Input: part model. Units: mm. Frame: model coordinates. A direction names the side the tool comes from. Give positions to 0.01 mm unless a question says otherwise; leave off trailing zeros. Write each loop counter-clockwise with the first axis right and the second up, starting at its lowest first coordinate (ties: lowest second). Pieces come first, ordered by that corner, then holes. Notation, with made-up numbers: (21, 65) - (52, 65) arc R33 cw to (52, 93) - close; hole circle Ø10 at (-21.75, 52). An arc over 180 degrees is marked (long way). Answer as CSV lines item,"result".
```python
from build123d import *

# Parameters (mm, degrees)
F0_W           = 12.7
F0_H           = 3.175
F1_DEPTH       = 6.35
F2_DEPTH       = 3.683
F4_DEPTH       = 30.48
F5_W           = 7.1628
F5_H           = 7.2898
F6_DEPTH       = 38.101
F3_W           = 6.731
F3_H           = 12.7
F7_DEPTH       = 11.43
F8_W           = 3.5814
F8_H           = 3.6449
F9_DEPTH       = 12.7
F11_DEPTH      = 11.43
F12_W          = 7.2898
F12_H          = 7.1628
F13_DEPTH      = 6.731
F13_DEPTH_BACK = 31.369
F14_W          = 7.2898
F14_H          = 7.1628
F15_DEPTH      = 6.731
F15_DEPTH_BACK = 31.369
F16_W          = 7.1628
F16_H          = 7.2898
F17_DEPTH      = 8.128
F18_DEPTH      = 8.128
F19_DEPTH      = 8.128
F20_W          = 11.43
F20_H          = 12.7
F20_W_2        = 7.1628
F20_H_2        = 7.2898
F21_DEPTH      = 8.128
F22_DEPTH      = 8.128
F23_DEPTH      = 8.128
F24_W          = 12.7
F24_H          = 11.43
F24_R          = 2.286
F25_DEPTH      = 2.032
F26_W          = 12.7
F26_H          = 11.43
F26_R          = 2.286
F27_DEPTH      = 2.032
F28_W          = 11.43
F28_H          = 12.7
F28_R          = 2.286
F29_DEPTH      = 2.032
F30_W          = 12.7
F30_H          = 11.43
F30_R          = 2.286
F31_DEPTH      = 2.032
F32_W          = 12.7
F32_H          = 11.43
F32_R          = 2.286
F33_DEPTH      = 2.032
F34_W          = 30.48
F34_H          = 12.7
F34_R          = 2.286
F35_DEPTH      = 2.032
F36_R          = 1.9533985806
F36_R_2        = 1.1294229331
F36_R_3        = 1.2624825339
F36_R_4        = 1.2356748077
F36_R_5        = 1.4795101848
F36_R_6        = 1.3424473069
F36_R_7        = 0.8820699454
F36_R_8        = 0.8709860762
F36_R_9        = 1.0254141301
F36_R_10       = 0.6987220166
F36_R_11       = 1.012521994
F36_W          = 3.4493412822
F36_H          = 0.7421383634
F36_W_2        = 3.1675938517
F36_H_2        = 1.3768810313
F36_W_3        = 3.0767889693
F36_H_3        = 1.3319775462
F37_DEPTH      = 0.508


with BuildPart() as f1:
    # F0 (on Front) → F1 (new body, symmetric)
    with BuildSketch(Plane.XZ):
        with BuildLine():
            Line((0, 3.175), (0, 0))
            Line((0, 0), (13.335, 0))
            ThreePointArc((13.335, 0), (19.6211792847, -2.6038207153), (22.225, -8.89))
            Line((22.225, -8.89), (22.225, -22.225))
            Line((22.225, -22.225), (25.4, -22.225))
            Line((25.4, -22.225), (25.4, 3.175))
            Line((25.4, 3.175), (0, 3.175))
        make_face()
        with BuildLine():
            Line((13.335, 0), (0, 0))
            Line((0, 0), (0, -3.556))
            Line((0, -3.556), (11.557, -3.556))
            ThreePointArc((11.557, -3.556), (16.5859434278, -5.6390565722), (18.669, -10.668))
            Line((18.669, -10.668), (18.669, -22.225))
            Line((18.669, -22.225), (22.225, -22.225))
            Line((22.225, -22.225), (22.225, -8.89))
            ThreePointArc((22.225, -8.89), (19.6211792847, -2.6038207153), (13.335, 0))
        make_face()
        with Locations((-6.35, 1.5875)):
            Rectangle(F0_W, F0_H)
        with BuildLine():
            Line((0, -3.556), (0, 0))
            Line((0, 0), (-12.7, 0))
            Line((-12.7, 0), (-12.7, -22.225))
            Line((-12.7, -22.225), (-5.969, -22.225))
            Line((-5.969, -22.225), (-5.969, -8.636))
            ThreePointArc((-5.969, -8.636), (-4.4811024484, -5.0438975516), (-0.889, -3.556))
            Line((-0.889, -3.556), (0, -3.556))
        make_face()
    extrude(amount=F1_DEPTH, both=True)

    # F0 (on Front) → F2 (cut, symmetric)
    with BuildSketch(Plane.XZ):
        with BuildLine():
            Line((13.335, 0), (0, 0))
            Line((0, 0), (0, -3.556))
            Line((0, -3.556), (11.557, -3.556))
            ThreePointArc((11.557, -3.556), (16.5859434278, -5.6390565722), (18.669, -10.668))
            Line((18.669, -10.668), (18.669, -22.225))
            Line((18.669, -22.225), (22.225, -22.225))
            Line((22.225, -22.225), (22.225, -8.89))
            ThreePointArc((22.225, -8.89), (19.6211792847, -2.6038207153), (13.335, 0))
        make_face()
        with BuildLine():
            Line((0, -3.556), (0, 0))
            Line((0, 0), (-12.7, 0))
            Line((-12.7, 0), (-12.7, -22.225))
            Line((-12.7, -22.225), (-5.969, -22.225))
            Line((-5.969, -22.225), (-5.969, -8.636))
            ThreePointArc((-5.969, -8.636), (-4.4811024484, -5.0438975516), (-0.889, -3.556))
            Line((-0.889, -3.556), (0, -3.556))
        make_face()
    extrude(amount=F2_DEPTH, both=True, mode=Mode.SUBTRACT)

    # F3 (on face) → F4 (join)
    with BuildSketch(Plane.XZ.offset(6.35)):
        Polygon((18.669, -10.668), (18.669, -22.225), (25.4, -22.225), (25.4, -9.525), (18.669, -9.525), align=None)
    extrude(amount=F4_DEPTH)

    # F5 (on face) → F6 (cut, through all)
    with BuildSketch(Plane.YZ.offset(25.4)):
        with Locations((-11.6205, -15.875)):
            Rectangle(F5_W, F5_H)
        with Locations((-21.1455, -15.875)):
            Rectangle(F5_W, F5_H)
        with Locations((-30.6705, -15.875)):
            Rectangle(F5_W, F5_H)
    extrude(amount=-F6_DEPTH, mode=Mode.SUBTRACT)

    # F3 (on face) → F7 (join)
    with BuildSketch(Plane.XZ.offset(6.35)):
        with Locations((-9.3345, -15.875)):
            Rectangle(F3_W, F3_H)
    extrude(amount=F7_DEPTH)

    # F8 (on face) → F9 (cut)
    with BuildSketch(Plane(origin=(-12.7, 0, 0), x_dir=(0, -1, 0), z_dir=(-1, 0, 0))):
        with Locations((13.4112, -14.05255)):
            Rectangle(F8_W, F8_H)
        with Locations((9.8298, -14.05255)):
            Rectangle(F8_W, F8_H)
        Polygon((15.2019, -19.5199), (15.2019, -15.875), (11.6205, -15.875), (8.0391, -15.875), (8.0391, -19.5199), align=None)
    extrude(amount=-F9_DEPTH, mode=Mode.SUBTRACT)

    # F10 (on face) → F11 (join, through all)
    with BuildSketch(Plane.XZ.offset(6.35)):
        Polygon((-5.969, -9.525), (-5.308761314, -8.3814330508), (5.689761314, -2.0314330508), (7.010238686, -2.0314330508), (18.008761314, -8.3814330508), (18.669, -9.525), (25.4, -9.525), (21.374261314, -2.5522160579), (10.375738686, 3.7977839421), (2.324261314, 3.7977839421), (-8.674261314, -2.5522160579), (-12.7, -9.525), align=None)
        Polygon((18.008761314, -23.3685669492), (7.010238686, -29.7185669492), (5.689761314, -29.7185669492), (-5.308761314, -23.3685669492), (-5.969, -22.225), (-12.7, -22.225), (-8.674261314, -29.1977839421), (2.324261314, -35.5477839421), (10.375738686, -35.5477839421), (21.374261314, -29.1977839421), (25.4, -22.225), (18.669, -22.225), align=None)
    extrude(amount=F11_DEPTH)

    # F12 (on face) → F13 (cut, two sides)
    with BuildSketch(Plane(origin=(2.3020766425, 0, -3.9873137078), x_dir=(0.8660254038, 0, 0.5), z_dir=(0.5, 0, -0.8660254038))) as f13_sk:
        with Locations((-2.438238686, 11.6205)):
            Rectangle(F12_W, F12_H)
    extrude(amount=-F13_DEPTH, mode=Mode.SUBTRACT)
    extrude(f13_sk.sketch, amount=F13_DEPTH_BACK, mode=Mode.SUBTRACT)

    # F14 (on face) → F15 (cut, two sides)
    with BuildSketch(Plane(origin=(0.8729233575, 0, 1.5119476062), x_dir=(0.8660254038, 0, -0.5), z_dir=(-0.5, 0, -0.8660254038))) as f15_sk:
        with Locations((13.436761314, 11.6205)):
            Rectangle(F14_W, F14_H)
    extrude(amount=-F15_DEPTH, mode=Mode.SUBTRACT)
    extrude(f15_sk.sketch, amount=F15_DEPTH_BACK, mode=Mode.SUBTRACT)

    # F16 (on face) → F17 (join)
    with BuildSketch(Plane.YZ.offset(25.4)):
        Polygon((-17.78, -9.525), (-36.83, -9.525), (-36.83, -22.225), (-17.78, -22.225), (-6.35, -22.225), (-6.35, -9.525), align=None)
        with Locations((-30.6705, -15.875)):
            Rectangle(F16_W, F16_H, mode=Mode.SUBTRACT)
        with Locations((-21.1455, -15.875)):
            Rectangle(F16_W, F16_H, mode=Mode.SUBTRACT)
        with Locations((-11.6205, -15.875)):
            Rectangle(F16_W, F16_H, mode=Mode.SUBTRACT)
    extrude(amount=F17_DEPTH)

    # F18 (add): a face of the model
    f18_faces = [f1.faces().sort_by_distance(p)[0] for p in [
        (21.2262913255, -12.065, -2.4667855452),
    ]]
    extrude(f18_faces, amount=F18_DEPTH)

    # F19 (add): a face of the model
    f19_faces = [f1.faces().sort_by_distance(p)[0] for p in [
        (2.1762913255, -12.065, 3.7123534294),
    ]]
    extrude(f19_faces, amount=F19_DEPTH)

    # F20 (on face) → F21 (join)
    with BuildSketch(Plane(origin=(-12.7, 0, 0), x_dir=(0, -1, 0), z_dir=(-1, 0, 0))):
        with Locations((12.065, -15.875)):
            Rectangle(F20_W, F20_H)
        with Locations((11.6205, -15.875)):
            Rectangle(F20_W_2, F20_H_2, mode=Mode.SUBTRACT)
    extrude(amount=F21_DEPTH)

    # F22 (add): a face of the model
    f22_faces = [f1.faces().sort_by_distance(p)[0] for p in [
        (-8.5262913255, -12.065, -29.2832144548),
    ]]
    extrude(f22_faces, amount=F22_DEPTH)

    # F23 (add): a face of the model
    f23_faces = [f1.faces().sort_by_distance(p)[0] for p in [
        (10.5237086745, -12.065, -35.4623534294),
    ]]
    extrude(f23_faces, amount=F23_DEPTH)

    # F24 (on face) → F25 (join)
    with BuildSketch(Plane(origin=(8.3024233575, 0, 14.3802190811), x_dir=(0.8660254038, 0, -0.5), z_dir=(0.5, 0, 0.8660254038))):
        with Locations((13.436761314, -12.065)):
            Rectangle(F24_W, F24_H)
        with Locations((13.436761314, -11.6205)):
            Circle(F24_R, mode=Mode.SUBTRACT)
    extrude(amount=F25_DEPTH)

    # F26 (on face) → F27 (join)
    with BuildSketch(Plane(origin=(-5.1274233575, 0, 8.880957767), x_dir=(0.8660254038, 0, 0.5), z_dir=(-0.5, 0, 0.8660254038))):
        with Locations((-2.438238686, -12.065)):
            Rectangle(F26_W, F26_H)
        with Locations((-2.4382386859, -11.6205)):
            Circle(F26_R, mode=Mode.SUBTRACT)
    extrude(amount=F27_DEPTH)

    # F28 (on face) → F29 (join)
    with BuildSketch(Plane(origin=(-20.828, 0, 0), x_dir=(0, -1, 0), z_dir=(-1, 0, 0))):
        with Locations((12.065, -15.875)):
            Rectangle(F28_W, F28_H)
        with Locations((11.6205, -15.875)):
            Circle(F28_R, mode=Mode.SUBTRACT)
    extrude(amount=F29_DEPTH)

    # F30 (on face) → F31 (join)
    with BuildSketch(Plane(origin=(-18.8755766425, 0, -32.693457767), x_dir=(0.8660254038, 0, -0.5), z_dir=(-0.5, 0, -0.8660254038))):
        with Locations((13.436761314, 12.065)):
            Rectangle(F30_W, F30_H)
        with Locations((13.436761314, 11.6205)):
            Circle(F30_R, mode=Mode.SUBTRACT)
    extrude(amount=F31_DEPTH)

    # F32 (on face) → F33 (join)
    with BuildSketch(Plane(origin=(22.0505766425, 0, -38.1927190811), x_dir=(0.8660254038, 0, 0.5), z_dir=(0.5, 0, -0.8660254038))):
        with Locations((-2.438238686, 12.065)):
            Rectangle(F32_W, F32_H)
        with Locations((-2.4382386859, 11.6205)):
            Circle(F32_R, mode=Mode.SUBTRACT)
    extrude(amount=F33_DEPTH)

    # F34 (on face) → F35 (join)
    with BuildSketch(Plane.YZ.offset(33.528)):
        with Locations((-21.59, -15.875)):
            Rectangle(F34_W, F34_H)
        with Locations((-30.6705, -15.875)):
            Circle(F34_R, mode=Mode.SUBTRACT)
        with Locations((-21.1455, -15.875)):
            Circle(F34_R, mode=Mode.SUBTRACT)
        with Locations((-11.6205, -15.875)):
            Circle(F34_R, mode=Mode.SUBTRACT)
    extrude(amount=F35_DEPTH)

    # F36 (on face) → F37 (join)
    with BuildSketch(Plane.XZ.offset(17.78)):
        with Locations((-17.4339655787, -15.3335016221)):
            Circle(F36_R)
        with Locations((-8.1460978836, 4.867112264)):
            Circle(F36_R_2)
        with Locations((-5.0520505756, 6.2466020445)):
            Circle(F36_R_3)
        with Locations((19.006319344, 6.5597151406)):
            Circle(F36_R_4)
        with Locations((15.3510505334, 4.5153293759)):
            Circle(F36_R_5)
        with Locations((19.4071084261, 2.9789232649)):
            Circle(F36_R_6)
        with Locations((19.83676292, -35.1207405329)):
            Circle(F36_R_7)
        with Locations((17.3755344003, -36.4661067724)):
            Circle(F36_R_8)
        with Locations((-7.1977977641, -37.3765304685)):
            Circle(F36_R_9)
        with Locations((-6.6677220166, -34.6863158047)):
            Circle(F36_R_10)
        with Locations((-4.3116188608, -35.7335619628)):
            Circle(F36_R_11)
        with Locations((-12.5252148136, -14.9380327202)):
            Rectangle(F36_W, F36_H)
        with Locations((16.394414939, 0.6884405157)):
            Rectangle(F36_W_2, F36_H_2)
        with Locations((17.0683967881, -32.4682071805)):
            Rectangle(F36_W_3, F36_H_3)
    extrude(amount=F37_DEPTH)


solid = f1.part
```
Item 1: Cut plane D-D on y = -1. Return the cut outline in (x, z) (3 decimals).
The answers:
outline,"(-12.7, 0) - (13.335, 0) arc R8.89 cw to (22.225, -8.89) - (22.225, -22.225) - (25.4, -22.225) - (25.4, 3.175) - (-12.7, 3.175) - close"
Item 2: Cut plane A-A on x = 28. Return the cut outline in (y, z) (3 decimals).
The answers:
outline,"(-36.83, -22.225) - (-6.35, -22.225) - (-6.35, -9.525) - (-36.83, -9.525) - close; hole (-34.252, -19.52) - (-27.089, -19.52) - (-27.089, -12.23) - (-34.252, -12.23) - close; hole (-24.727, -19.52) - (-17.564, -19.52) - (-17.564, -12.23) - (-24.727, -12.23) - close; hole (-15.202, -19.52) - (-8.039, -19.52) - (-8.039, -12.23) - (-15.202, -12.23) - close"
Item 3: Cut plane B-B on y = -5.5. Return the cut outline in (x, z) (3 decimals).
The answers:
outline,"(-12.7, -22.225) - (-5.969, -22.225) - (-5.969, -8.636) arc R5.08 cw to (-0.889, -3.556) - (11.557, -3.556) arc R7.112 cw to (18.669, -10.668) - (18.669, -22.225) - (25.4, -22.225) - (25.4, 3.175) - (-12.7, 3.175) - close"
Item 4: Reachability of faces 4 (the face through (-17, -18.288, -15)), 5 (the face through (-20.828, -10, -14)), 6 (the face through (-2, -6.35, -6)), 7 (the face through (-9, 5, -22.225)) from +Z, -Z, +X, -X, +Y, -Y: full face, straight path, thin tool, end or side. Return the list, or none.
The answers:
face 4,"+Z, -Z, -X, -Y"
face 5,"none"
face 6,"-Z, +Y"
face 7,"-Z, +X, -X, +Y"
Item 5: Ray query, line 1 (Z direction, x = 30, y = -24) (3 decimals); line 2 (Y direction, x = -5, z = 8.5); line 3 (Y direction, x = 7, z = -2). Return the intervals inside material, ascending. Write a range as from..to.
The answers:
line 1,"-22.225..-19.52, -12.23..-9.525"
line 2,"-17.78..-15.2, -8.04..-6.35"
line 3,"-17.78..-3.68, 3.68..6.35"
Item 6: Cut plane C-C on y = -20. Return the cut outline in (x, z) (3 decimals).
The answers:
outline,"(18.669, -22.225) - (35.56, -22.225) - (35.56, -17.853) - (33.528, -17.853) - (33.528, -19.52) - (18.669, -19.52) - close; (18.669, -12.23) - (33.528, -12.23) - (33.528, -13.897) - (35.56, -13.897) - (35.56, -9.525) - (18.669, -9.525) - close"
Item 7: Mould query, pull axis X, two halves, no side actions, for faces 1 (the face through (34.53, -10.566, -17.903)), 2 (the face through (-13, -12, -12.23)), 3 (the face through (19.69, -0.052, -2.673)). Classes: +X half, -X half, draft (parallel to the pull), parting line (faces both ways), or undercut.
The answers:
face 1,"draft"
face 2,"undercut"
face 3,"-X half"
Item 8: Contact query for flat-ended pins moving along their axis: pin 1 (2 mm diameter, centred on x = 25.5, z = -27.5, fed in from +Y); pin 2 (13.5 mm diameter, centred on x = 29.5, y = -26, fed in from -Z) (3 decimals); pin 3 (1.5 mm diameter, centred on x = 16, z = 1, fed in from -Y); pin 4 (1 mm diameter, centred on x = 15.5, z = -25.5, fed in from +Y). Output: stop coordinate, or through.
The answers:
pin 1,"through"
pin 2,"z = -22.225"
pin 3,"y = -18.29"
pin 4,"y = -6.35"
